from build123d import *

# Parameters (mm, degrees)
SKETCH1_W           = 139.7
SKETCH1_H           = 63.5
BOSS_EXTRUDE1_DEPTH = 6.35
SKETCH2_R           = 1.778
CUT_EXTRUDE1_DEPTH  = 6.35
SKETCH3_R           = 2.413
CUT_EXTRUDE2_DEPTH  = 6.35


with BuildPart() as part:
    # Sketch1 → Boss-Extrude1 (new body)
    with BuildSketch(Plane.XY):
        with Locations((69.85, 31.75)):
            Rectangle(SKETCH1_W, SKETCH1_H)
    extrude(amount=BOSS_EXTRUDE1_DEPTH)

    # Sketch2 → Cut-Extrude1 (cut)
    with BuildSketch(Plane(origin=(0, 0, 0), x_dir=(-1, 0, 0), z_dir=(0, 0, -1))):
        with Locations((-65.024, 13.15775)):
            Circle(SKETCH2_R)
        with Locations((-65.024, 51.25775)):
            Circle(SKETCH2_R)
    extrude(amount=-CUT_EXTRUDE1_DEPTH, mode=Mode.SUBTRACT)

    # Sketch3 → Cut-Extrude2 (cut)
    with BuildSketch(Plane(origin=(0, 0, 0), x_dir=(-1, 0, 0), z_dir=(0, 0, -1))):
        with Locations((-111.865, 7.1)):
            Circle(SKETCH3_R)
        with Locations((-101.995, 7.1)):
            Circle(SKETCH3_R)
        with Locations((-111.865, 56.4)):
            Circle(SKETCH3_R)
        with Locations((-101.995, 56.4)):
            Circle(SKETCH3_R)
        with Locations((-37.705, 56.4)):
            Circle(SKETCH3_R)
        with Locations((-27.835, 56.4)):
            Circle(SKETCH3_R)
        with Locations((-27.835, 7.1)):
            Circle(SKETCH3_R)
        with Locations((-37.705, 7.1)):
            Circle(SKETCH3_R)
    extrude(amount=-CUT_EXTRUDE2_DEPTH, mode=Mode.SUBTRACT)


solid = part.part
Design review of the part built by this model. Coordinates are the model's own, in mm. Coordinates: 2 decimals unless noted, no trailing zeros. Loops run counter-clockwise (first coordinate to the right, second up) from the corner with the lowest first, then second, coordinate; pieces in that order, holes last. Notation, with made-up numbers: (26, 50) -> (66, 50) arc R14 cw to (66, 61) -> close; hole circle Ø11 at (48.25, -10). An arc over 180 degrees is marked (long way). Use a Markdown table: item, result. Add a question column.
Item 1: We need section B-B, the plane z = 1.75. Count the separate pieces of the cut face and the enclosed holes in it, and give its area (3 significant figures).
Item 2: Wall thickness on L1, parallel to Y at x = 104, z = 4.5; L2, parallel to X at y = 57.5, z = 3.25: over which ranges is each line inside the solid? List them lowest first. Write a range as from..to.
Item 3: The part is to be moulded in two halves that separate along Y. For faces 1 (the flat face through (139.7, 31, 3)), 2 (the cylindrical face through (63.38, 50.58, 3.13)), 3 (the flat face through (69, 63.5, 3)), say which applies: +Y half, -Y half, draft (parallel to the pull), parting line (faces both ways), or undercut.
Item 4: We need section A-A, the plane y = 7.1. Write out the cut boundary in (x, z), and give its area (3 significant figures).
Numbers:
| question | item | result |
|---|---|---|
| 1 | separate pieces | 1 |
| 1 | enclosed holes | 10 |
| 1 | area | 8,700 mm^2 |
| 2 | L1 | y = 0..5.76, 8.44..55.06, 57.74..63.5 |
| 2 | L2 | x = 0..25.69, 29.98..35.56, 39.85..99.85, 104.14..109.72, 114.01..139.7 |
| 3 | face 1 | draft |
| 3 | face 2 | undercut |
| 3 | face 3 | +Y half |
| 4 | outline | (0, 0) -> (25.42, 0) -> (25.42, 6.35) -> (0, 6.35) -> close; (30.25, 0) -> (35.29, 0) -> (35.29, 6.35) -> (30.25, 6.35) -> close; (40.12, 0) -> (99.58, 0) -> (99.58, 6.35) -> (40.12, 6.35) -> close; (104.41, 0) -> (109.45, 0) -> (109.45, 6.35) -> (104.41, 6.35) -> close; (114.28, 0) -> (139.7, 0) -> (139.7, 6.35) -> (114.28, 6.35) -> close |
| 4 | area | 765 mm^2 |
